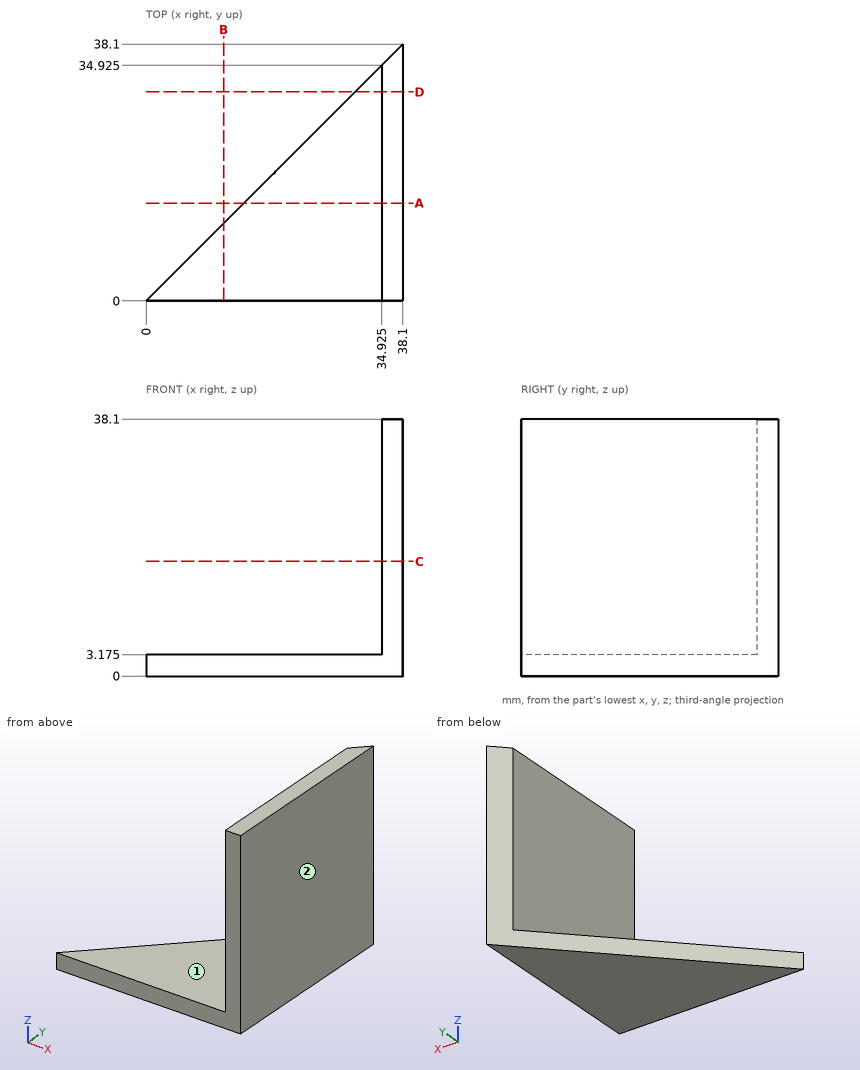
Can you work these out from the drawing? Everything is in mm from the part's minimum corner. A direction names the side the tool comes from. Coordinates: 2 decimals unless noted, no trailing zeros. Loops run counter-clockwise (first coordinate to the right, second up) from the corner with the lowest first, then second, coordinate; pieces in that order, holes last.
1. Imagine slicing it at A-A, the plane y = 14.5. Please give me the cut outline in (x, z) (3 decimals).
2. For the marked faces 1 and 2, which set-ups out of +Z, -Z, +X, -X, +Y, -Y let a thin tool reach every point of the face, with its end or its side?
3. For P1, Ø4, axis at x = 23, y = 23.5, coming from the +Z side (3 decimals); P2, Ø1.5, axis at x = 12, z = 5.5, coming from the +Y side; P3, Ø8, axis at y = 7, z = 12.5, coming from the -X side (3 decimals), each with a flat end and sliding along its axis, tell me the tip position at first contact or that it passes through.
4. Imagine slicing it at C-C, the plane z = 17. Please give me the cut outline in (x, y) (3 decimals), and give its area (3 significant figures).
5. Imagine slicing it at D-D, the plane y = 31. Please give me the cut outline in (x, z) (3 decimals).
6. Imagine slicing it at B-B, the plane x = 11.5. Please give me the cut outline in (y, z) (3 decimals), and give its area (3 significant figures).
7. I need wall thicknesses on L1, parallel to X at y = 31.5, z = 21.5 (3 decimals); L2, parallel to Z at x = 32.5, y = 13.5 (3 decimals); L3, parallel to X at y = 33, z = 2.5. Which ranges of each line are inside material? Lowest first, please.
Taken from the geometry:
1. outline: (14.5, 0) - (38.1, 0) - (38.1, 38.1) - (34.925, 38.1) - (34.925, 3.175) - (14.5, 3.175) - close
2. face 1: +Z, -X, +Y, -Y
2. face 2: +Z, -Z, +X, +Y, -Y
3. P1: stops at z = 3.175
3. P2: passes through
3. P3: stops at x = 34.925
4. outline: (34.925, 0) - (38.1, 0) - (38.1, 38.1) - (34.925, 34.925) - close
4. area: 116 mm2
5. outline: (31, 0) - (38.1, 0) - (38.1, 38.1) - (34.925, 38.1) - (34.925, 3.175) - (31, 3.175) - close
6. outline: (0, 0) - (11.5, 0) - (11.5, 3.175) - (0, 3.175) - close
6. area: 36.5 mm2
7. L1: x = 34.925 to 38.1
7. L2: z = 0 to 3.175
7. L3: x = 33 to 38.1
